```python
from build123d import *

# Parameters (mm, degrees)
SKETCH2_W          = 84
SKETCH2_H          = 84
CUT_EXTRUDE1_DEPTH = 6


with BuildPart() as part:
    # Sketch1 → Revolve1 (revolve)
    with BuildSketch(Plane.XY, mode=Mode.PRIVATE) as revolve1_sk:
        with BuildLine():
            Line((0, 21), (0, 6))
            Line((0, 6), (47, 6))
            Line((47, 6), (47, 9.45))
            ThreePointArc((47, 9.45), (46.69246212, 10.19246212), (45.95, 10.5))
            Line((45.95, 10.5), (7, 10.5))
            Line((7, 10.5), (7, 10.2))
            Line((7, 10.2), (6, 10.2))
            Line((6, 10.2), (6, 21))
            Line((6, 21), (0, 21))
        make_face()
    revolve(revolve1_sk.sketch.rotate(Axis((47, 0, 0), (-1, 0, 0)), 270), axis=Axis((47, 0, 0), (-1, 0, 0)))

    # Sketch2 → Cut-Extrude1 (cut)
    with BuildSketch(Plane(origin=(0, 0, 0), x_dir=(0, 0, -1), z_dir=(1, 0, 0))):
        Rectangle(SKETCH2_W, SKETCH2_H)
        with BuildLine():
            Line((13.5, -16.085707942), (13.5, 16.085707942))
            ThreePointArc((13.5, 16.085707942), (0, 21), (-13.5, 16.085707942))
            Line((-13.5, 16.085707942), (-13.5, -16.085707942))
            ThreePointArc((-13.5, -16.085707942), (0, -21), (13.5, -16.085707942))
        make_face(mode=Mode.SUBTRACT)
    extrude(amount=CUT_EXTRUDE1_DEPTH, mode=Mode.SUBTRACT)

    # Sketch3 → Cut-Revolve1 (revolve, cut)
    with BuildSketch(Plane.XY, mode=Mode.PRIVATE) as cut_revolve1_sk:
        Polygon((0, 16), (0, 19.75), (4.1, 19.75), (4.1, 18.25), (6, 18.25), (6, 16), align=None)
    revolve(cut_revolve1_sk.sketch.rotate(Axis((6, 16, 0), (-1, 0, 0)), 270), axis=Axis((6, 16, 0), (-1, 0, 0)), mode=Mode.SUBTRACT)

    # Sketch4 → Cut-Revolve2 (revolve, cut)
    with BuildSketch(Plane.XY, mode=Mode.PRIVATE) as cut_revolve2_sk:
        Polygon((0, -16), (0, -12.25), (4.1, -12.25), (4.1, -13.75), (6, -13.75), (6, -16), align=None)
    revolve(cut_revolve2_sk.sketch.rotate(Axis((6, -16, 0), (-1, 0, 0)), 270), axis=Axis((6, -16, 0), (-1, 0, 0)), mode=Mode.SUBTRACT)


solid = part.part
```
Could you check a few things on this model? Use its own coordinates, in mm. A direction names the side the tool comes from. Give positions to 0.01 mm unless a question says otherwise; leave off trailing zeros. Order: outer loops, then holes, each group sorted by start corner. A loop starts at its lowest first (then second) coordinate and runs counter-clockwise, first axis right, second up.
Q1. If I drill on line 1 along Y through (x, z) = (1.65, 0); line 2 along Y through (x, z) = (4.95, 0); line 3 along Y through (x, z) = (15, 0), over which ranges is the centre line in solid material (lowest first)?
Q2. Suppose I cut it at B-B, the plane y = 0. Write out the boundary of the cut face in (x, z), and give its area (3 significant figures).
Q3. Suppose I cut it at D-D, the plane y = -17.5. Write out the boundary of the cut face in (x, z), and give its area (3 significant figures).
Q4. We'd pull the mould along Y, two halves only. Please class faces 4 (the flat face through (4.1, 14, 2)), 5 (the cylindrical face through (2.08, 12.34, -0.81)), 6 (the flat face through (0, 0.3, -6.2)), 7 (the cylindrical face through (3, 21, 0)): +Y half, -Y half, draft (parallel to the pull), parting line (faces both ways), or undercut.
Q5. For faces 1 (the cylindrical face through (26.2, 3.2, 10)), 2 (the flat face through (4.1, -18, 2)), 3 (the cylindrical face through (6.49, 3.06, 9.73)), which set-ups out of +Z, -Z, +X, -X, +Y, -Y let a thin tool reach every point of the face, with its end or its side?
Q6. Suppose I cut it at A-A, the plane z = 0. Count the separate pieces of the cut face and the enclosed holes in it, and give its area (3 significant figures).
Q7. Suppose I cut it at C-C, the plane x = 5. Write out the boundary of the cut face in (y, z), and give its area (3 significant figures).
Q8. I'm going to push flat-ended pins straight in: P1, Ø3, axis at x = 36, y = -6, coming from the -Z side; P2, Ø1, axis at x = 40, y = -4, coming from the +Z side; P3, Ø8, axis at x = 20.5, z = -2.5, coming from the -Y side. Where does each tip first touch, or does it pass through?
Solution:
1. line 1: y = -21 to -19.75, -12.25 to -6, 6 to 12.25, 19.75 to 21
1. line 2: y = -21 to -18.25, -13.75 to -6, 6 to 13.75, 18.25 to 21
1. line 3: y = -10.5 to -6, 6 to 10.5
2. outline: (0, -13.5) - (6, -13.5) - (6, -10.2) - (7, -10.2) - (7, -10.5) - (45.95, -10.5) arc R1.05 ccw to (47, -9.45) - (47, -6) - (0, -6) - close; (0, 6) - (47, 6) - (47, 9.45) arc R1.05 ccw to (45.95, 10.5) - (7, 10.5) - (7, 10.2) - (6, 10.2) - (6, 13.5) - (0, 13.5) - close
2. area: 458 mm2
3. outline: (0, -11.61) - (6, -11.61) - (6, -1.68) - (4.1, -1.68) - (4.1, -3.44) - (0, -3.44) - close; (0, 3.44) - (4.1, 3.44) - (4.1, 1.68) - (6, 1.68) - (6, 11.61) - (0, 11.61) - close
3. area: 105 mm2
4. face 4: undercut
4. face 5: undercut
4. face 6: draft
4. face 7: +Y half
5. face 1: +X
5. face 2: -X
5. face 3: none
6. separate pieces: 4
6. enclosed holes: 0
6. area: 469 mm2
7. outline: (-16.09, -13.5) - (16.09, -13.5) arc R21 ccw to (16.09, 13.5) - (-16.09, 13.5) arc R21 ccw to start; hole circle Ø4.5 at (-16, 0); hole circle Ø12 at (0, 0); hole circle Ø4.5 at (16, 0)
7. area: 905 mm2
8. P1: stops at z = -9.49
8. P2: stops at z = 9.9
8. P3: stops at y = -10.5
